For this review, take the finished solid that the model builds, in its own axes (mm). A direction names the side the tool comes from. Coordinates: 2 decimals unless noted, no trailing zeros. Loops run counter-clockwise (first coordinate to the right, second up) from the corner with the lowest first, then second, coordinate; pieces in that order, holes last. Notation, with made-up numbers: (84.5, 66) - (90.5, 66) arc R20 ccw to (90.5, 82) - close; hole circle Ø11 at (75.25, -15). An arc over 180 degrees is marked (long way). One line per item, written item: value. Start each with the question number.
1. The part is to be moulded in two halves that separate along Y. For faces 4 (the face through (-14.248, -19.814, 41.374)), 5 (the face through (13.976, -0.632, 0.986)), 6 (the face through (-17.074, 0.496, 0.986)), say which applies: released by +Y, released by -Y, zero draft, split by the parting line, or undercut.
2. To check wall thickness, follow line 1 (Y direction, x = -1, z = 13.5); line 2 (Z direction, x = -11, y = 9.5); line 3 (Z direction, x = 7, y = -19). State the ranges of each line that lie inside material, in increasing order. Write a range as from..to.
3. Insertion check: pin 1 (12 mm diameter, centred on x = 5, z = 7, fed in from +Y); pin 2 (4.5 mm diameter, centred on x = 15.6, z = 14.3, fed in from +Y); pin 3 (4 mm diameter, centred on x = -7.75, y = -13.42, fed in from +Z). Each pin has a flat end and moves straight along its axis. Give the tip position at first contact, or say it passes through.
4. For faces 1 (the face through (8, -4, 2)), 2 (the face through (-15.512, -19.814, 22.698)), 3 (the face through (-6.6, 0, 1)), list the 3-axis set-ups (+Z, -Z, +X, -X, +Y, -Y) from which the entire face can be reached by the end or side of a thin tool; tool diameter is ignored.
5. Take a section at B-B, the plane y = 9. State the section outline as (x, z) points, and give its area (3 significant figures).
6. Take a section at D-D, the plane z = 21.5. State the section outline as (x, y) points.
7. Take a section at A-A, the plane z = 27.1. State the section outline as (x, y) points, and give its area (3 significant figures).
8. Take a section at C-C, the plane x = -3. State the section outline as (y, z) points.
```python
from build123d import *

# Parameters (mm, degrees)
BOSS_EXTRUDE1_DEPTH = 2
SKETCH2_W           = 37.6
SKETCH2_H           = 2
BOSS_EXTRUDE2_DEPTH = 49.2
FILLET1_R           = 2
FILLET2_R           = 3
CUT_EXTRUDE1_REACH  = 69.402
SKETCH3_R           = 2
CUT_EXTRUDE2_REACH  = 60.374
SKETCH4_R           = 1.65


with BuildPart() as part:
    # Sketch1 → Boss-Extrude1 (new body)
    with BuildSketch(Plane.XY):
        with BuildLine():
            Line((-18.8, 0), (-18.8, -20.8))
            Line((-18.8, -20.8), (18.8, -20.8))
            Line((18.8, -20.8), (18.8, 0))
            ThreePointArc((18.8, 0), (0, 18.8), (-18.8, 0))
        make_face()
    extrude(amount=BOSS_EXTRUDE1_DEPTH)

    # Sketch2 → Boss-Extrude2 (add)
    with BuildSketch(Plane.XY.offset(2)):
        with Locations((0, -19.8)):
            Rectangle(SKETCH2_W, SKETCH2_H)
    extrude(amount=BOSS_EXTRUDE2_DEPTH)

    # Fillet1
    fillet1_edges = [part.edges().sort_by_distance(p)[0] for p in [
        (0, -20.8, 0),
    ]]
    fillet(fillet1_edges, radius=FILLET1_R)

    # Fillet2
    fillet2_edges = [part.edges().sort_by_distance(p)[0] for p in [
        (-18.8, -19.8, 51.2),
        (18.8, -19.8, 51.2),
    ]]
    fillet(fillet2_edges, radius=FILLET2_R)

    # Sketch3 → Cut-Extrude1 (cut, up to next)
    with BuildSketch(Plane.XZ.offset(20.8), mode=Mode.PRIVATE) as cut_extrude1_sk1:
        with Locations(Location((-15.6, 46.3, 0), (0, 0, 270))):
            Circle(SKETCH3_R)
    cut_extrude1_tool1 = extrude(cut_extrude1_sk1.sketch, amount=-CUT_EXTRUDE1_REACH, mode=Mode.PRIVATE) & part.part
    # Sketch3 → Cut-Extrude1 (cut, up to next)
    with BuildSketch(Plane.XZ.offset(20.8), mode=Mode.PRIVATE) as cut_extrude1_sk2:
        with Locations(Location((15.6, 46.3, 0), (0, 0, 270))):
            Circle(SKETCH3_R)
    cut_extrude1_tool2 = extrude(cut_extrude1_sk2.sketch, amount=-CUT_EXTRUDE1_REACH, mode=Mode.PRIVATE) & part.part
    # Sketch3 → Cut-Extrude1 (cut, up to next)
    with BuildSketch(Plane.XZ.offset(20.8), mode=Mode.PRIVATE) as cut_extrude1_sk3:
        with Locations(Location((-15.6, 39.9, 0), (0, 0, 270))):
            Circle(SKETCH3_R)
    cut_extrude1_tool3 = extrude(cut_extrude1_sk3.sketch, amount=-CUT_EXTRUDE1_REACH, mode=Mode.PRIVATE) & part.part
    # Sketch3 → Cut-Extrude1 (cut, up to next)
    with BuildSketch(Plane.XZ.offset(20.8), mode=Mode.PRIVATE) as cut_extrude1_sk4:
        with Locations(Location((15.6, 39.9, 0), (0, 0, 270))):
            Circle(SKETCH3_R)
    cut_extrude1_tool4 = extrude(cut_extrude1_sk4.sketch, amount=-CUT_EXTRUDE1_REACH, mode=Mode.PRIVATE) & part.part
    # Sketch3 → Cut-Extrude1 (cut, up to next)
    with BuildSketch(Plane.XZ.offset(20.8), mode=Mode.PRIVATE) as cut_extrude1_sk5:
        with Locations(Location((-15.6, 33.5, 0), (0, 0, 270))):
            Circle(SKETCH3_R)
    cut_extrude1_tool5 = extrude(cut_extrude1_sk5.sketch, amount=-CUT_EXTRUDE1_REACH, mode=Mode.PRIVATE) & part.part
    # Sketch3 → Cut-Extrude1 (cut, up to next)
    with BuildSketch(Plane.XZ.offset(20.8), mode=Mode.PRIVATE) as cut_extrude1_sk6:
        with Locations(Location((15.6, 33.5, 0), (0, 0, 270))):
            Circle(SKETCH3_R)
    cut_extrude1_tool6 = extrude(cut_extrude1_sk6.sketch, amount=-CUT_EXTRUDE1_REACH, mode=Mode.PRIVATE) & part.part
    # Sketch3 → Cut-Extrude1 (cut, up to next)
    with BuildSketch(Plane.XZ.offset(20.8), mode=Mode.PRIVATE) as cut_extrude1_sk7:
        with Locations(Location((-15.6, 27.1, 0), (0, 0, 270))):
            Circle(SKETCH3_R)
    cut_extrude1_tool7 = extrude(cut_extrude1_sk7.sketch, amount=-CUT_EXTRUDE1_REACH, mode=Mode.PRIVATE) & part.part
    # Sketch3 → Cut-Extrude1 (cut, up to next)
    with BuildSketch(Plane.XZ.offset(20.8), mode=Mode.PRIVATE) as cut_extrude1_sk8:
        with Locations(Location((15.6, 27.1, 0), (0, 0, 270))):
            Circle(SKETCH3_R)
    cut_extrude1_tool8 = extrude(cut_extrude1_sk8.sketch, amount=-CUT_EXTRUDE1_REACH, mode=Mode.PRIVATE) & part.part
    # Sketch3 → Cut-Extrude1 (cut, up to next)
    with BuildSketch(Plane.XZ.offset(20.8), mode=Mode.PRIVATE) as cut_extrude1_sk9:
        with Locations(Location((-15.6, 20.7, 0), (0, 0, 270))):
            Circle(SKETCH3_R)
    cut_extrude1_tool9 = extrude(cut_extrude1_sk9.sketch, amount=-CUT_EXTRUDE1_REACH, mode=Mode.PRIVATE) & part.part
    # Sketch3 → Cut-Extrude1 (cut, up to next)
    with BuildSketch(Plane.XZ.offset(20.8), mode=Mode.PRIVATE) as cut_extrude1_sk10:
        with Locations(Location((15.6, 20.7, 0), (0, 0, 270))):
            Circle(SKETCH3_R)
    cut_extrude1_tool10 = extrude(cut_extrude1_sk10.sketch, amount=-CUT_EXTRUDE1_REACH, mode=Mode.PRIVATE) & part.part
    # Sketch3 → Cut-Extrude1 (cut, up to next)
    with BuildSketch(Plane.XZ.offset(20.8), mode=Mode.PRIVATE) as cut_extrude1_sk11:
        with Locations(Location((-15.6, 14.3, 0), (0, 0, 270))):
            Circle(SKETCH3_R)
    cut_extrude1_tool11 = extrude(cut_extrude1_sk11.sketch, amount=-CUT_EXTRUDE1_REACH, mode=Mode.PRIVATE) & part.part
    # Sketch3 → Cut-Extrude1 (cut, up to next)
    with BuildSketch(Plane.XZ.offset(20.8), mode=Mode.PRIVATE) as cut_extrude1_sk12:
        with Locations(Location((15.6, 14.3, 0), (0, 0, 270))):
            Circle(SKETCH3_R)
    cut_extrude1_tool12 = extrude(cut_extrude1_sk12.sketch, amount=-CUT_EXTRUDE1_REACH, mode=Mode.PRIVATE) & part.part
    # Sketch3 → Cut-Extrude1 (cut, up to next)
    with BuildSketch(Plane.XZ.offset(20.8), mode=Mode.PRIVATE) as cut_extrude1_sk13:
        with Locations(Location((-15.6, 7.9, 0), (0, 0, 270))):
            Circle(SKETCH3_R)
    cut_extrude1_tool13 = extrude(cut_extrude1_sk13.sketch, amount=-CUT_EXTRUDE1_REACH, mode=Mode.PRIVATE) & part.part
    # Sketch3 → Cut-Extrude1 (cut, up to next)
    with BuildSketch(Plane.XZ.offset(20.8), mode=Mode.PRIVATE) as cut_extrude1_sk14:
        with Locations(Location((15.6, 7.9, 0), (0, 0, 270))):
            Circle(SKETCH3_R)
    cut_extrude1_tool14 = extrude(cut_extrude1_sk14.sketch, amount=-CUT_EXTRUDE1_REACH, mode=Mode.PRIVATE) & part.part
    add(cut_extrude1_tool1.solids().sort_by_distance((-15.6, -20.8, 46.3))[0], mode=Mode.SUBTRACT)
    add(cut_extrude1_tool2.solids().sort_by_distance((15.6, -20.8, 46.3))[0], mode=Mode.SUBTRACT)
    add(cut_extrude1_tool3.solids().sort_by_distance((-15.6, -20.8, 39.9))[0], mode=Mode.SUBTRACT)
    add(cut_extrude1_tool4.solids().sort_by_distance((15.6, -20.8, 39.9))[0], mode=Mode.SUBTRACT)
    add(cut_extrude1_tool5.solids().sort_by_distance((-15.6, -20.8, 33.5))[0], mode=Mode.SUBTRACT)
    add(cut_extrude1_tool6.solids().sort_by_distance((15.6, -20.8, 33.5))[0], mode=Mode.SUBTRACT)
    add(cut_extrude1_tool7.solids().sort_by_distance((-15.6, -20.8, 27.1))[0], mode=Mode.SUBTRACT)
    add(cut_extrude1_tool8.solids().sort_by_distance((15.6, -20.8, 27.1))[0], mode=Mode.SUBTRACT)
    add(cut_extrude1_tool9.solids().sort_by_distance((-15.6, -20.8, 20.7))[0], mode=Mode.SUBTRACT)
    add(cut_extrude1_tool10.solids().sort_by_distance((15.6, -20.8, 20.7))[0], mode=Mode.SUBTRACT)
    add(cut_extrude1_tool11.solids().sort_by_distance((-15.6, -20.8, 14.3))[0], mode=Mode.SUBTRACT)
    add(cut_extrude1_tool12.solids().sort_by_distance((15.6, -20.8, 14.3))[0], mode=Mode.SUBTRACT)
    add(cut_extrude1_tool13.solids().sort_by_distance((-15.6, -20.8, 7.9))[0], mode=Mode.SUBTRACT)
    add(cut_extrude1_tool14.solids().sort_by_distance((15.6, -20.8, 7.9))[0], mode=Mode.SUBTRACT)

    # Sketch4 → Cut-Extrude2 (cut, up to next)
    with BuildSketch(Plane(origin=(0, 0, 0), x_dir=(-1, 0, 0), z_dir=(0, 0, -1)), mode=Mode.PRIVATE) as cut_extrude2_sk1:
        with Locations((15.5, 0)):
            Circle(SKETCH4_R)
    cut_extrude2_tool1 = extrude(cut_extrude2_sk1.sketch, amount=-CUT_EXTRUDE2_REACH, mode=Mode.PRIVATE) & part.part
    # Sketch4 → Cut-Extrude2 (cut, up to next)
    with BuildSketch(Plane(origin=(0, 0, 0), x_dir=(-1, 0, 0), z_dir=(0, 0, -1)), mode=Mode.PRIVATE) as cut_extrude2_sk2:
        with Locations((7.75, -13.423393759)):
            Circle(SKETCH4_R)
    cut_extrude2_tool2 = extrude(cut_extrude2_sk2.sketch, amount=-CUT_EXTRUDE2_REACH, mode=Mode.PRIVATE) & part.part
    # Sketch4 → Cut-Extrude2 (cut, up to next)
    with BuildSketch(Plane(origin=(0, 0, 0), x_dir=(-1, 0, 0), z_dir=(0, 0, -1)), mode=Mode.PRIVATE) as cut_extrude2_sk3:
        with Locations((-7.75, -13.423393759)):
            Circle(SKETCH4_R)
    cut_extrude2_tool3 = extrude(cut_extrude2_sk3.sketch, amount=-CUT_EXTRUDE2_REACH, mode=Mode.PRIVATE) & part.part
    # Sketch4 → Cut-Extrude2 (cut, up to next)
    with BuildSketch(Plane(origin=(0, 0, 0), x_dir=(-1, 0, 0), z_dir=(0, 0, -1)), mode=Mode.PRIVATE) as cut_extrude2_sk4:
        with Locations((-15.5, 0)):
            Circle(SKETCH4_R)
    cut_extrude2_tool4 = extrude(cut_extrude2_sk4.sketch, amount=-CUT_EXTRUDE2_REACH, mode=Mode.PRIVATE) & part.part
    # Sketch4 → Cut-Extrude2 (cut, up to next)
    with BuildSketch(Plane(origin=(0, 0, 0), x_dir=(-1, 0, 0), z_dir=(0, 0, -1)), mode=Mode.PRIVATE) as cut_extrude2_sk5:
        with Locations((-7.75, 13.423393759)):
            Circle(SKETCH4_R)
    cut_extrude2_tool5 = extrude(cut_extrude2_sk5.sketch, amount=-CUT_EXTRUDE2_REACH, mode=Mode.PRIVATE) & part.part
    # Sketch4 → Cut-Extrude2 (cut, up to next)
    with BuildSketch(Plane(origin=(0, 0, 0), x_dir=(-1, 0, 0), z_dir=(0, 0, -1)), mode=Mode.PRIVATE) as cut_extrude2_sk6:
        with Locations((7.75, 13.423393759)):
            Circle(SKETCH4_R)
    cut_extrude2_tool6 = extrude(cut_extrude2_sk6.sketch, amount=-CUT_EXTRUDE2_REACH, mode=Mode.PRIVATE) & part.part
    # Sketch4 → Cut-Extrude2 (cut, up to next)
    with BuildSketch(Plane(origin=(0, 0, 0), x_dir=(-1, 0, 0), z_dir=(0, 0, -1)), mode=Mode.PRIVATE) as cut_extrude2_sk7:
        with BuildLine():
            Line((-6.6, 7), (-6.6, -7))
            ThreePointArc((-6.6, -7), (0, -13.6), (6.6, -7))
            Line((6.6, -7), (6.6, 7))
            ThreePointArc((6.6, 7), (0, 13.6), (-6.6, 7))
        make_face()
    cut_extrude2_tool7 = extrude(cut_extrude2_sk7.sketch, amount=-CUT_EXTRUDE2_REACH, mode=Mode.PRIVATE) & part.part
    add(cut_extrude2_tool1.solids().sort_by_distance((-15.5, 0, 0))[0], mode=Mode.SUBTRACT)
    add(cut_extrude2_tool2.solids().sort_by_distance((-7.75, -13.423394, 0))[0], mode=Mode.SUBTRACT)
    add(cut_extrude2_tool3.solids().sort_by_distance((7.75, -13.423394, 0))[0], mode=Mode.SUBTRACT)
    add(cut_extrude2_tool4.solids().sort_by_distance((15.5, 0, 0))[0], mode=Mode.SUBTRACT)
    add(cut_extrude2_tool5.solids().sort_by_distance((7.75, 13.423394, 0))[0], mode=Mode.SUBTRACT)
    add(cut_extrude2_tool6.solids().sort_by_distance((-7.75, 13.423394, 0))[0], mode=Mode.SUBTRACT)
    add(cut_extrude2_tool7.solids().sort_by_distance((0, 0, 0))[0], mode=Mode.SUBTRACT)


solid = part.part
```
Solutions:
1. face 4: zero draft
1. face 5: undercut
1. face 6: undercut
2. line 1: -20.8..-18.8
2. line 2: 0..2
2. line 3: 0.01..51.2
3. pin 1: y = 18.72
3. pin 2: y = -18.8
3. pin 3: z = 2
4. face 1: +Z, +X, -X, +Y
4. face 2: +Y, -Y
4. face 3: +Z, -Z
5. outline: (-16.51, 0) - (-6.29, 0) - (-6.29, 2) - (-16.51, 2) - close; (6.29, 0) - (16.51, 0) - (16.51, 2) - (6.29, 2) - close
5. area: 40.9 mm2
6. outline: (-18.8, -20.8) - (-17.43, -20.8) - (-17.43, -18.8) - (-18.8, -18.8) - close; (-13.77, -20.8) - (13.77, -20.8) - (13.77, -18.8) - (-13.77, -18.8) - close; (17.43, -20.8) - (18.8, -20.8) - (18.8, -18.8) - (17.43, -18.8) - close
7. outline: (-18.8, -20.8) - (-17.6, -20.8) - (-17.6, -18.8) - (-18.8, -18.8) - close; (-13.6, -20.8) - (13.6, -20.8) - (13.6, -18.8) - (-13.6, -18.8) - close; (17.6, -20.8) - (18.8, -20.8) - (18.8, -18.8) - (17.6, -18.8) - close
7. area: 59.2 mm2
8. outline: (-20.8, 2) arc R2 ccw to (-18.8, 0) - (-12.88, 0) - (-12.88, 2) - (-18.8, 2) - (-18.8, 51.2) - (-20.8, 51.2) - close; (12.88, 0) - (18.56, 0) - (18.56, 2) - (12.88, 2) - close
